Build history of the part. All positions in model axes, mm. Face numbers are marked on the shaded views. A direction names the side the tool comes from. Coordinates: 2 decimals unless noted, no trailing zeros. Loops run counter-clockwise (first coordinate to the right, second up) from the corner with the lowest first, then second, coordinate; pieces in that order, holes last. Notation, with made-up numbers: M 18.25,-15.75 L 48.25,-15.75 A35 cw 48.25,23.25 Z; hole C -1.75,20 d7. An arc over 180 degrees is marked long. Write each question's results on one line, items separated by ' | '. Start each with the question number.
from build123d import *

# Parameters (mm, degrees)
SKETCH1_W           = 88.9
SKETCH1_H           = 50.8
BOSS_EXTRUDE1_DEPTH = 68.58
SHELL10_T           = 3
SKETCH4_W           = 62.58
SKETCH4_H           = 44.8
CUT_EXTRUDE2_DEPTH  = 10
SKETCH2_R           = 6
SKETCH2_R_2         = 1.6
SKETCH2_W           = 22.9
SKETCH2_H           = 44.8
CUT_EXTRUDE3_DEPTH  = 68.59
SKETCH5_R           = 18.3
CUT_EXTRUDE4_DEPTH  = 62.58
CUT_EXTRUDE7_START  = -1.5
SKETCH10_R          = 6
SKETCH10_R_2        = 1.6
CUT_EXTRUDE7_DEPTH  = 1.5
SKETCH10_8_R        = 6
SKETCH10_8_R_2      = 1.6
CUT_EXTRUDE8_DEPTH  = 64.08
SKETCH12_W          = 15.003225859
SKETCH12_H          = 62.579342489
CUT_EXTRUDE9_DEPTH  = 3


with BuildPart() as part:
    # Sketch1 → Boss-Extrude1 (new body)
    with BuildSketch(Plane.XY):
        with Locations((44.45, 25.4)):
            Rectangle(SKETCH1_W, SKETCH1_H)
    extrude(amount=BOSS_EXTRUDE1_DEPTH)

    # Shell10 (no face opened: a closed hollow body)
    add(offset(amount=-SHELL10_T, mode=Mode.PRIVATE), mode=Mode.SUBTRACT)

    # Sketch4 → Cut-Extrude2 (cut)
    with BuildSketch(Plane.ZY):
        with Locations((34.29, 25.4)):
            Rectangle(SKETCH4_W, SKETCH4_H)
    extrude(amount=-CUT_EXTRUDE2_DEPTH, mode=Mode.SUBTRACT)

    # Sketch2 → Cut-Extrude3 (cut)
    with BuildSketch(Plane.XY.offset(68.58)):
        with Locations(Location((25, 19, 0), (0, 0, 180))):
            Circle(SKETCH2_R)
        with Locations(Location((4, 19, 0), (0, 0, 180))):
            Circle(SKETCH2_R_2)
        with Locations(Location((46, 19, 0), (0, 0, 180))):
            Circle(SKETCH2_R_2)
        with Locations((74.45, 25.4)):
            Rectangle(SKETCH2_W, SKETCH2_H)
    extrude(amount=-CUT_EXTRUDE3_DEPTH, mode=Mode.SUBTRACT)

    # Sketch5 → Cut-Extrude4 (cut)
    with BuildSketch(Plane(origin=(0, 0, 65.58), x_dir=(-1, 0, 0), z_dir=(0, 0, -1))):
        with Locations((-25, 19)):
            Circle(SKETCH5_R)
    extrude(amount=CUT_EXTRUDE4_DEPTH, mode=Mode.SUBTRACT)

    # Sketch10 → Cut-Extrude7 (cut)
    # profile 1 of 5: a face of its own
    with BuildSketch(Plane(origin=(0, 0, 65.58), x_dir=(-1, 0, 0), z_dir=(0, 0, -1)).offset(CUT_EXTRUDE7_START)):
        with BuildLine():
            ThreePointArc((-39.966629547, 9), (-25, 1), (-10.033370453, 9))
            Line((-10.033370453, 9), (-39.966629547, 9))
        make_face()
    # profile 2 of 5: a face of its own
    with BuildSketch(Plane(origin=(0, 0, 65.58), x_dir=(-1, 0, 0), z_dir=(0, 0, -1)).offset(CUT_EXTRUDE7_START)):
        with BuildLine():
            Line((-39.966629547, 9), (-10.033370453, 9))
            ThreePointArc((-10.033370453, 9), (-7.77502784, 13.77502784), (-7, 19))
            ThreePointArc((-7, 19), (-7.77502784, 24.22497216), (-10.033370453, 29))
            Line((-10.033370453, 29), (-39.966629547, 29))
            ThreePointArc((-39.966629547, 29), (-43, 19), (-39.966629547, 9))
        make_face()
        with Locations(Location((-25, 19, 0), (0, 0, 180))):
            Circle(SKETCH10_R, mode=Mode.SUBTRACT)
    # profile 3 of 5: a face of its own
    with BuildSketch(Plane(origin=(0, 0, 65.58), x_dir=(-1, 0, 0), z_dir=(0, 0, -1)).offset(CUT_EXTRUDE7_START)):
        with BuildLine():
            Line((-39.966629547, 29), (-10.033370453, 29))
            ThreePointArc((-10.033370453, 29), (-25, 37), (-39.966629547, 29))
        make_face()
    # profile 4 of 5: a face of its own
    with BuildSketch(Plane(origin=(0, 0, 65.58), x_dir=(-1, 0, 0), z_dir=(0, 0, -1)).offset(CUT_EXTRUDE7_START)):
        with BuildLine():
            Line((-50, 9), (-39.966629547, 9))
            ThreePointArc((-39.966629547, 9), (-43, 19), (-39.966629547, 29))
            Line((-39.966629547, 29), (-50, 29))
            Line((-50, 29), (-50, 9))
        make_face()
        with Locations(Location((-46, 19, 0), (0, 0, 180))):
            Circle(SKETCH10_R_2, mode=Mode.SUBTRACT)
    # profile 5 of 5: a face of its own
    with BuildSketch(Plane(origin=(0, 0, 65.58), x_dir=(-1, 0, 0), z_dir=(0, 0, -1)).offset(CUT_EXTRUDE7_START)):
        with BuildLine():
            Line((-10.033370453, 9), (0, 9))
            Line((0, 9), (0, 29))
            Line((0, 29), (-10.033370453, 29))
            ThreePointArc((-10.033370453, 29), (-7.77502784, 24.22497216), (-7, 19))
            ThreePointArc((-7, 19), (-7.77502784, 13.77502784), (-10.033370453, 9))
        make_face()
        with Locations(Location((-4, 19, 0), (0, 0, 180))):
            Circle(SKETCH10_R_2, mode=Mode.SUBTRACT)
    extrude(amount=CUT_EXTRUDE7_DEPTH, mode=Mode.SUBTRACT)

    # Sketch10_8 → Cut-Extrude8 (cut)
    # profile 1 of 5: a face of its own
    with BuildSketch(Plane(origin=(0, 0, 65.58), x_dir=(-1, 0, 0), z_dir=(0, 0, -1))):
        with BuildLine():
            ThreePointArc((-39.966629547, 9), (-25, 1), (-10.033370453, 9))
            Line((-10.033370453, 9), (-39.966629547, 9))
        make_face()
    # profile 2 of 5: a face of its own
    with BuildSketch(Plane(origin=(0, 0, 65.58), x_dir=(-1, 0, 0), z_dir=(0, 0, -1))):
        with BuildLine():
            Line((-39.966629547, 9), (-10.033370453, 9))
            ThreePointArc((-10.033370453, 9), (-7.77502784, 13.77502784), (-7, 19))
            ThreePointArc((-7, 19), (-7.77502784, 24.22497216), (-10.033370453, 29))
            Line((-10.033370453, 29), (-39.966629547, 29))
            ThreePointArc((-39.966629547, 29), (-43, 19), (-39.966629547, 9))
        make_face()
        with Locations(Location((-25, 19, 0), (0, 0, 180))):
            Circle(SKETCH10_8_R, mode=Mode.SUBTRACT)
    # profile 3 of 5: a face of its own
    with BuildSketch(Plane(origin=(0, 0, 65.58), x_dir=(-1, 0, 0), z_dir=(0, 0, -1))):
        with BuildLine():
            Line((-10.033370453, 9), (0, 9))
            Line((0, 9), (0, 29))
            Line((0, 29), (-10.033370453, 29))
            ThreePointArc((-10.033370453, 29), (-7.77502784, 24.22497216), (-7, 19))
            ThreePointArc((-7, 19), (-7.77502784, 13.77502784), (-10.033370453, 9))
        make_face()
        with Locations(Location((-4, 19, 0), (0, 0, 180))):
            Circle(SKETCH10_8_R_2, mode=Mode.SUBTRACT)
    # profile 4 of 5: a face of its own
    with BuildSketch(Plane(origin=(0, 0, 65.58), x_dir=(-1, 0, 0), z_dir=(0, 0, -1))):
        with BuildLine():
            Line((-39.966629547, 29), (-10.033370453, 29))
            ThreePointArc((-10.033370453, 29), (-25, 37), (-39.966629547, 29))
        make_face()
    # profile 5 of 5: a face of its own
    with BuildSketch(Plane(origin=(0, 0, 65.58), x_dir=(-1, 0, 0), z_dir=(0, 0, -1))):
        with BuildLine():
            Line((-50, 9), (-39.966629547, 9))
            ThreePointArc((-39.966629547, 9), (-43, 19), (-39.966629547, 29))
            Line((-39.966629547, 29), (-50, 29))
            Line((-50, 29), (-50, 9))
        make_face()
        with Locations(Location((-46, 19, 0), (0, 0, 180))):
            Circle(SKETCH10_8_R_2, mode=Mode.SUBTRACT)
    extrude(amount=CUT_EXTRUDE8_DEPTH, mode=Mode.SUBTRACT)

    # Sketch12 → Cut-Extrude9 (cut)
    with BuildSketch(Plane(origin=(0, 50.8, 0), x_dir=(1, 0, 0), z_dir=(0, 1, 0))):
        with Locations((16.393449041, -34.290328755)):
            Rectangle(SKETCH12_W, SKETCH12_H)
    extrude(amount=-CUT_EXTRUDE9_DEPTH, mode=Mode.SUBTRACT)


solid = part.part
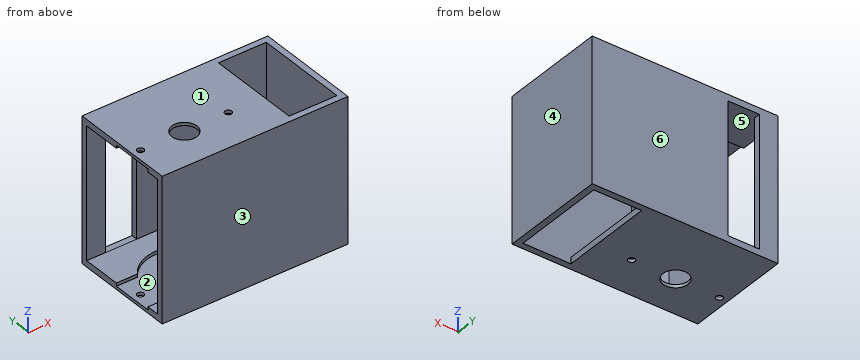
1. Band-saw the part on B-B, the plane z = 8.5. List the corners of the cut face in (x, y).
2. Band-saw the part on D-D, the plane x = 38. List the corners of the cut face in (y, z).
3. Band-saw the part on A-A, the plane x = 4. List the corners of the cut face in (y, z).
4. Which spindle directions (+Z, -Z, +X, -X, +Y, -Y) get a long thin tool onto all of the face, cutting with end or side? Do the marked faces 1 and 2. Say none if no direction does.
5. Band-saw the part on C-C, the plane y = 46. List the corners of the cut face in (x, z).
6. Pin check, flat tips, straight feed: pin 1 (7 mm diameter, centred on x = 25, y = 19, fed in from -Z); pin 2 (12 mm diameter, centred on y = 25, z = 43.5, fed in from -X); pin 3 (0.8 mm diameter, centred on y = 20, z = 2, fed in from -X). Stop position of each tip, or through.
7. Wall check: line 1 along Z through (x, y) = (37, 17.5); line 2 along Y through (x, z) = (5.5, 62.5); line 3 along X through (y, z) = (19, 68.35). Give the ranges that are in metal, low to high.
8. Mould opens along Y. For the marked faces 3, 4, 5 and 6 say: +Y half, -Y half, draft (parallel to the pull), parting line (faces both ways), or undercut.
Checked values:
1) outline: M 0,0 L 88.9,0 L 88.9,50.8 L 23.9,50.8 L 23.9,47.8 L 85.9,47.8 L 85.9,3 L 33.88,3 A18.3 cw 16.12,3 L 0,3 Z; M 0,47.8 L 8.89,47.8 L 8.89,50.8 L 0,50.8 Z
2) outline: M 0,0 L 50.8,0 L 50.8,68.58 L 0,68.58 Z; hole M 3,3 L 6.55,3 L 6.55,1.5 L 31.45,1.5 L 31.45,3 L 47.8,3 L 47.8,65.58 L 31.45,65.58 L 31.45,67.08 L 6.55,67.08 L 6.55,65.58 L 3,65.58 Z
3) outline: M 0,0 L 17.4,0 L 17.4,1.5 L 9,1.5 L 9,3 L 3,3 L 3,65.58 L 9,65.58 L 9,67.08 L 17.4,67.08 L 17.4,68.58 L 0,68.58 Z; M 20.6,0 L 50.8,0 L 50.8,68.58 L 20.6,68.58 L 20.6,67.08 L 29,67.08 L 29,65.58 L 47.8,65.58 L 47.8,3 L 29,3 L 29,1.5 L 20.6,1.5 Z
4) face 1: +Z, +X, -X, +Y, -Y | face 2: none
5) outline: M 0,0 L 63,0 L 63,3 L 0,3 Z; M 0,65.58 L 63,65.58 L 63,68.58 L 0,68.58 Z; M 85.9,0 L 88.9,0 L 88.9,68.58 L 85.9,68.58 Z
6) pin 1: through | pin 2: x = 85.9 | pin 3: x = 50
7) line 1: 0 to 1.5, 67.08 to 68.58 | line 2: 0 to 3, 47.8 to 50.8 | line 3: 0 to 2.4, 5.6 to 19, 31 to 44.4, 47.6 to 63, 85.9 to 88.9
8) face 3: -Y half | face 4: draft | face 5: undercut | face 6: +Y half
